CAD build for the part. Positions are in the model's coordinates, mm. A direction names the side the tool comes from. Round coordinates to 2 decimals unless told otherwise and drop trailing zeros. Loops run counter-clockwise (first coordinate to the right, second up) from the corner with the lowest first, then second, coordinate; pieces in that order, holes last. Notation, with made-up numbers: M 20.25,-26.75 L 36.25,-26.75 A9 ccw 36.25,-17.75 Z; hole C 38.25,14.5 d9. An arc over 180 degrees is marked long. Put each result on its own line as item: value. Start each with the question number.
from build123d import *

# Parameters (mm, degrees)
PAD002_DEPTH = 8
SKETCH_R     = 3
PAD_DEPTH    = 3
FILLET_R     = 2.75


with BuildPart() as part:
    # Sketch002 → Pad002 (new body)
    with BuildSketch(Plane.XZ.offset(-2)):
        Polygon((20, 0.5), (20, 2.5), (-10, 2.5), (-10, 0.547361), (-10, -3), (-4, -3), (-4, -1), (-8, -1), (-8, 0.5), align=None)
    extrude(amount=PAD002_DEPTH)

    # Sketch (on Face2 of Pad002) → Pad (join)
    with BuildSketch(Plane(origin=(0, 2, 2.5), x_dir=(-1, 0, 0), z_dir=(0, 0, 1))):
        with Locations((-10, 4)):
            Circle(SKETCH_R)
    extrude(amount=PAD_DEPTH)

    # Fillet
    fillet_edges = [part.edges().sort_by_distance(p)[0] for p in [
        (13, -2, 5.5),
    ]]
    fillet(fillet_edges, radius=FILLET_R)


solid = part.part
(1) Tool access for faces 1 (the flat face through (-4, -2, -2)), 2 (the flat face through (20, -2, 1)): list every direction of +Z, -Z, +X, -X, +Y, -Y with a clear straight run to the whole face (end or side of a thin tool).
(2) Mould opens along Z. For faces 3 (the flat face through (1, 2, 1)), 4 (the flat face through (-6, -2, -1)), 5 (the flat face through (-7, -2, -3)), 6 (the flat face through (-8, -2, 0)) say: +Z half, -Z half, draft (parallel to the pull), parting line (faces both ways), or undercut.
(3) Cut at C-C on x = 15.25. List the corners of the cut face in (y, z).
(4) Drill centre lines: line 1 along Z through (x, y) = (-4.5, -0.75); line 2 along X through (y, z) = (-1.5, -1.5); line 3 along Z through (x, y) = (4, -2.5). Where is each one in solid material? Low to high.
(5) Cut at B-B on z = -1.75. List the corners of the cut face in (x, y), and give its area (3 significant figures).
(6) Flat gauge pins, fed straight in: pin 1 Ø3 at (x, y) = (-6, -2.5) entering from +Z; pin 2 Ø0.6 at (y, z) = (-1.5, -2) entering from +X; pin 3 Ø2 at (y, z) = (-3, 0) entering from +X; pin 4 Ø0.8 at (y, z) = (-0.5, 0) entering from +X. Where does each tip first touch, or does it go through?
(7) Cut at A-A on y = 1.5. List the corners of the cut face in (x, z).
Taken from the geometry:
1. face 1: -Z, +X, +Y, -Y
1. face 2: +Z, -Z, +X, +Y, -Y
2. face 3: draft
2. face 4: undercut
2. face 5: -Z half
2. face 6: undercut
3. outline: M -6,0.5 L 2,0.5 L 2,2.5 L -6,2.5 Z
4. line 1: -3 to -1, 0.5 to 2.5
4. line 2: -10 to -4
4. line 3: 0.5 to 2.5
5. outline: M -10,-6 L -4,-6 L -4,2 L -10,2 Z
5. area: 48.0 mm2
6. pin 1: z = 2.5
6. pin 2: x = -4
6. pin 3: x = 20
6. pin 4: x = -8
7. outline: M -10,-3 L -4,-3 L -4,-1 L -8,-1 L -8,0.5 L 20,0.5 L 20,2.5 L -10,2.5 Z
